Geometry: final body of the model. Coordinates: model frame, mm. A direction names the side the tool comes from. Give positions to 0.01 mm unless a question says otherwise; leave off trailing zeros. Loops run counter-clockwise (first coordinate to the right, second up) from the corner with the lowest first, then second, coordinate; pieces in that order, holes last. Notation, with made-up numbers: M 30,30 L 86,30 A20 ccw 86,46 Z; hole C -7.75,61.25 d11. An arc over 180 degrees is marked long. Put each result on its own line as item: value.
```python
from build123d import *

# Parameters (mm, degrees)
F1_DEPTH = 25
F2_DEPTH = 12.5


with BuildPart() as f1:
    # F0 (on Front) → F1 (new body, symmetric)
    with BuildSketch(Plane.XZ):
        with BuildLine():
            Line((-2.408674, -10.917151), (-4.461097, -6.113606))
            Line((-4.461097, -6.113606), (-5.875311, -4.699392))
            Line((-5.875311, -4.699392), (-11.532165, 0.957462))
            Line((-11.532165, 0.957462), (108.011199, 11.416151))
            Line((108.011199, 11.416151), (156.30749, 24.357103))
            ThreePointArc((156.30749, 24.357103), (157.014597, 25.581849), (155.789852, 26.288956))
            Line((155.789852, 26.288956), (107.662575, 13.393291))
            Line((107.662575, 13.393291), (-11.619487, 2.957463))
            Line((-11.619487, 2.957463), (-22.568457, 2.957463))
            Line((-22.568457, 2.957463), (-41.653733, -3.478072))
            Line((-41.653733, -3.478072), (-22.568462, -9.913606))
            Line((-22.568462, -9.913606), (-22.568462, -11.613606))
            Line((-22.568462, -11.613606), (-2.868462, -11.613606))
            ThreePointArc((-2.868462, -11.613606), (-2.451193, -11.38908), (-2.408674, -10.917151))
        make_face()
    extrude(amount=F1_DEPTH, both=True)

    # F0 (on Front) → F2 (join, symmetric)
    with BuildSketch(Plane.XZ):
        Polygon((-11.532165, 0.957462), (-5.875311, -4.699392), (108.011199, 11.416151), align=None)
    extrude(amount=F2_DEPTH, both=True)


solid = f1.part
```
Item 1: Set-up query: faces 1 (the flat face through (-17, 0, 2.957)), 2 (the flat face through (-3.42, -0.35, -8.55)), 3 (the flat face through (-32.245, -0.35, -6.651)). Return all of +Z, -Z, +X, -X, +Y, -Y with unobstructed straight access to the full face (end or side cutting, diameter ignored); none if empty.
Output values:
face 1: +Z, -X, +Y, -Y
face 2: +X, +Y, -Y
face 3: -Z, -X, +Y, -Y
Item 2: Section D-D on y = 0. Output: boundary loops of the cut face in (x, z).
Output values:
outline: M -41.65,-3.48 L -22.57,-9.91 L -22.57,-11.61 L -2.87,-11.61 A0.5 ccw -2.41,-10.92 L -4.46,-6.11 L -5.88,-4.7 L 108.01,11.42 L 156.31,24.36 A1 ccw 155.79,26.29 L 107.66,13.39 L -11.62,2.96 L -22.57,2.96 Z
Item 3: Section A-A on y = 21.5. Output: boundary loops of the cut face in (x, z), then the cut area to 3 significant figures.
Output values:
outline: M -41.65,-3.48 L -22.57,-9.91 L -22.57,-11.61 L -2.87,-11.61 A0.5 ccw -2.41,-10.92 L -4.46,-6.11 L -11.53,0.96 L 108.01,11.42 L 156.31,24.36 A1 ccw 155.79,26.29 L 107.66,13.39 L -11.62,2.96 L -22.57,2.96 Z
area: 695 mm²
Item 4: Section B-B on x = 86. Output: boundary loops of the cut face in (y, z), then the cut area to 3 significant figures.
Output values:
outline: M -25,9.49 L -12.5,9.49 L -12.5,8.3 L 12.5,8.3 L 12.5,9.49 L 25,9.49 L 25,11.5 L -25,11.5 Z
area: 130 mm²
Item 5: Section C-C on z = 9. Output: boundary loops of the cut face in (x, y).
Output values:
outline: M 57.45,-25 L 80.39,-25 L 80.39,-12.5 L 90.94,-12.5 L 90.94,12.5 L 80.39,12.5 L 80.39,25 L 57.45,25 Z
Item 6: Line query: probe 1 along Z at (x, y) = (-13, -11.5); probe 2 along Z at (x, y) = (-31, -5). Output: solid intervals per line, ascending. Write a range as [from, to].
Output values:
probe 1: [-11.61, 2.96]
probe 2: [-7.07, 0.11]
Item 7: Pin query (flat end, axial travel): pin 1 Ø2 at (x, y) = (33.5, -9) entering from -Z; pin 2 Ø8 at (x, y) = (104, -7) entering from +Z; pin 3 Ø9 at (x, y) = (-16, 0.5) entering from +Z; pin 4 Ø3 at (x, z) = (2.5, 6) entering from -Y. Return the tip coordinate at first contact, or that it passes through.
Output values:
pin 1: z = 0.73
pin 2: z = 13.48
pin 3: z = 2.97
pin 4: through
